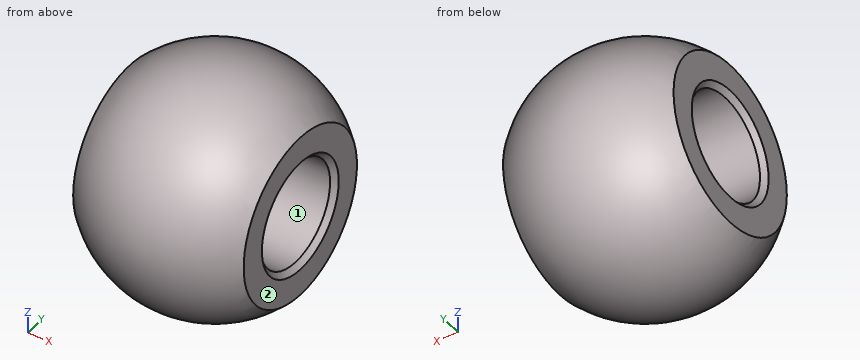
from build123d import *

# Parameters (mm, degrees)
SKETCH2_R               = 2.38125
CUT_EXTRUDE1_DEPTH      = 6.5372
CUT_EXTRUDE1_DEPTH_BACK = 6.5372
CUT_EXTRUDE2_START      = 3.96875
SKETCH3_R               = 5
CUT_EXTRUDE2_DEPTH      = 2.030273132
CHAMFER1_SIZE           = 0.23876


with BuildPart() as part:
    # Sketch1 → Revolve1 (revolve)
    with BuildSketch(Plane.XY):
        with BuildLine():
            Line((0, 5.5372), (0, -5.5372))
            ThreePointArc((0, -5.5372), (-5.5372, 0), (0, 5.5372))
        make_face()
    revolve(axis=Axis((0, 5.5372, 0), (0, -1, 0)))

    # Sketch2 → Cut-Extrude1 (cut, two sides)
    with BuildSketch(Plane(origin=(0, 0, 0), x_dir=(0, 0, -1), z_dir=(1, 0, 0))) as cut_extrude1_sk:
        Circle(SKETCH2_R)
    extrude(amount=CUT_EXTRUDE1_DEPTH, mode=Mode.SUBTRACT)
    extrude(cut_extrude1_sk.sketch, amount=-CUT_EXTRUDE1_DEPTH_BACK, mode=Mode.SUBTRACT)

    # Sketch3 → Cut-Extrude2 (cut, through all)
    with BuildSketch(Plane(origin=(0, 0, 0), x_dir=(0, 0, -1), z_dir=(1, 0, 0)).offset(CUT_EXTRUDE2_START)):
        Circle(SKETCH3_R)
    cut_extrude2 = extrude(amount=CUT_EXTRUDE2_DEPTH, mode=Mode.SUBTRACT)

    # Mirror1: Cut-Extrude2 across plane
    add(cut_extrude2.mirror(Plane(origin=(0, 0, 0), x_dir=(0, 0, 1), z_dir=(1, 0, 0))), mode=Mode.SUBTRACT)

    # Chamfer1
    chamfer1_edges = [part.edges().sort_by_distance(p)[0] for p in [
        (3.96875, 0, 2.38125),
        (-3.96875, 0, 2.38125),
    ]]
    chamfer(chamfer1_edges, length=CHAMFER1_SIZE)


solid = part.part
Check sheet for the modelled part. Datum: model origin and axes. Units: mm. Face numbers are marked on the shaded views. Coordinates: 2 decimals unless noted, no trailing zeros. Loops run counter-clockwise (first coordinate to the right, second up) from the corner with the lowest first, then second, coordinate; pieces in that order, holes last. Notation, with made-up numbers: (-36.75, 5) -> (1.25, 5) arc R16 ccw to (1.25, 13) -> close; hole circle Ø5 at (0, 36.25). An arc over 180 degrees is marked (long way). Answer in a Markdown table with one row per item.
1. Sectioned sample at D-D, the plane y = -3.5. Record the boundary of the cut face in (x, z).
Check values:
| item | result |
|---|---|
| outline | (-3.97, -1.63) arc R4.29 ccw to (3.97, -1.63) -> (3.97, 1.63) arc R4.29 ccw to (-3.97, 1.63) -> close |
2. Sectioned sample at A-A, the plane y = 0. Record the boundary of the cut face in (x, z).
Check values:
| item | result |
|---|---|
| outline | (-3.97, -3.86) arc R5.54 ccw to (3.97, -3.86) -> (3.97, -2.62) -> (3.73, -2.38) -> (-3.73, -2.38) -> (-3.97, -2.62) -> close; (-3.97, 2.62) -> (-3.73, 2.38) -> (3.73, 2.38) -> (3.97, 2.62) -> (3.97, 3.86) arc R5.54 ccw to (-3.97, 3.86) -> close |
3. Go/stop test with flat-tipped pins: pin 1 (1.5 mm diameter, centred on y = -3.5, z = 4, fed in from -X); pin 2 (2 mm diameter, centred on x = -1, z = 1, fed in from +Y); pin 3 (4 mm diameter, centred on x = 3, y = 2.5, fed in from -Z). Record where each tip stops, or that it passes through.
Check values:
| item | result |
|---|---|
| pin 1 | stops at x = -3.13 |
| pin 2 | stops at y = 5.52 |
| pin 3 | stops at z = -5.2 |
4. Material ranges on line 1 along Z through (x, y) = (2.5, -0.25); line 2 along Z through (x, y) = (-1.75, 2); line 3 along Y through (x, z) = (0.25, 0), recorded low to high. Write a range as [from, to].
Check values:
| item | result |
|---|---|
| line 1 | z = [-4.93, -2.37], [2.37, 4.93] |
| line 2 | z = [-4.86, -1.29], [1.29, 4.86] |
| line 3 | y = [-5.53, -2.38], [2.38, 5.53] |
5. Release check for a two-part mould opening along Y. For the marked faces 1 and 2 record: released by +Y, released by -Y, zero draft, split by the parting line, or undercut.
Check values:
| item | result |
|---|---|
| face 1 | undercut |
| face 2 | zero draft |
6. Sectioned sample at C-C, the plane x = 0.25. Record the boundary of the cut face in (y, z), then the cut area to 3 significant figures.
Check values:
| item | result |
|---|---|
| outline | circle Ø11.06 at (0, 0); hole circle Ø4.76 at (0, 0) |
| area | 78.3 mm2 |
